Check sheet for the modelled part. Datum: model origin and axes. Units: mm. A direction names the side the tool comes from. Coordinates: 2 decimals unless noted, no trailing zeros. Order: outer loops, then holes, each group sorted by start corner. A loop starts at its lowest first (then second) coordinate and runs counter-clockwise, first axis right, second up. Notation, with made-up numbers: (42, 11.5) -> (89, 11.5) arc R26 ccw to (89, 26.5) -> close; hole circle Ø10 at (9, -31.75). An arc over 180 degrees is marked (long way). Put each result on its own line as item: value. Start each with the question number.
```python
from build123d import *

# Parameters (mm, degrees)
F0_W     = 57.15
F0_H     = 63.5
F1_DEPTH = 44.45
F2_W     = 22.225
F2_H     = 19.05
F3_DEPTH = 12.7
F4_W     = 19.05
F4_H     = 12.7
F5_DEPTH = 63.501


with BuildPart() as f1:
    # F0 (on Front) → F1 (new body)
    with BuildSketch(Plane.XZ):
        Rectangle(F0_W, F0_H)
    extrude(amount=F1_DEPTH)

    # F2 (on face) → F3 (join)
    with BuildSketch(Plane(origin=(0, 0, 0), x_dir=(-1, 0, 0), z_dir=(0, 1, 0))):
        with Locations((-39.6875, -22.225)):
            Rectangle(F2_W, F2_H)
    extrude(amount=-F3_DEPTH)

    # F4 (on face) → F5 (cut, through all)
    with BuildSketch(Plane.XY.offset(31.75)):
        with Locations((3.175, -38.1)):
            Rectangle(F4_W, F4_H)
    extrude(amount=-F5_DEPTH, mode=Mode.SUBTRACT)


solid = f1.part
```
1) Mould release check, pull along X, two halves, no side actions. Record for faces 4 (the flat face through (12.7, -38, 0)), 5 (the flat face through (50.8, -6, -22)), 6 (the flat face through (21, -44.45, 0)), 7 (the flat face through (-6.35, -38, 0)): +X half, -X half, draft (parallel to the pull), parting line (faces both ways), or undercut.
2) Sectioned sample at D-D (x = 32.5). Record the boundary of the cut face in (y, z).
3) Scan lines: line 1 along X through (y, z) = (-36, -24) (3 decimals); line 2 along X through (y, z) = (-28.5, -16.5) (3 decimals); line 3 along Y through (x, z) = (-5, -1). Record each from-to range of solid material in increasing order. Write a range as [from, to].
4) Gauge pin test, flat ends, axial feed: pin 1 (9.5 mm diameter, centred on x = 0.5, z = -4.5, fed in from -Y); pin 2 (3 mm diameter, centred on x = 30.5, y = -32, fed in from +Z); pin 3 (1 mm diameter, centred on y = -33, z = -13.5, fed in from +X) (3 decimals); pin 4 (14 mm diameter, centred on x = 39.5, y = -5.5, fed in from +Z). Record the tip position at first contact, or that the pin passes through.
5) Sectioned sample at B-B (z = 7). Record the boundary of the cut face in (x, y) (3 decimals).
6) Access from +Z, -Z, +X, -X, +Y, -Y to the whole of each face (thin tool, end or side, straight path). Record for faces 1 (the flat face through (40, -12.7, -22)), 2 (the flat face through (3, -31.75, 0)), 3 (the flat face through (40, -6, -12.7)).
7) Sectioned sample at C-C (y = -6). Record the boundary of the cut face in (x, z) (3 decimals), plus the area to 3 significant figures.
8) Sectioned sample at A-A (y = -33). Record the boundary of the cut face in (x, z) (3 decimals), plus the area to 3 significant figures.
Entries:
1. face 4: undercut
1. face 5: +X half
1. face 6: draft
1. face 7: undercut
2. outline: (-12.7, -31.75) -> (0, -31.75) -> (0, -12.7) -> (-12.7, -12.7) -> close
3. line 1: x = [-28.575, -6.35], [12.7, 28.575]
3. line 2: x = [-28.575, 28.575]
3. line 3: y = [-31.75, 0]
4. pin 1: stops at y = -31.75
4. pin 2: passes through
4. pin 3: stops at x = 28.575
4. pin 4: stops at z = -12.7
5. outline: (-28.575, -44.45) -> (-6.35, -44.45) -> (-6.35, -31.75) -> (12.7, -31.75) -> (12.7, -44.45) -> (28.575, -44.45) -> (28.575, 0) -> (-28.575, 0) -> close
6. face 1: +Z, -Z, +X, -Y
6. face 2: +Z, -Z, -Y
6. face 3: +Z, +X, +Y, -Y
7. outline: (-28.575, -31.75) -> (50.8, -31.75) -> (50.8, -12.7) -> (28.575, -12.7) -> (28.575, 31.75) -> (-28.575, 31.75) -> close
7. area: 4,050 mm2
8. outline: (-28.575, -31.75) -> (-6.35, -31.75) -> (-6.35, 31.75) -> (-28.575, 31.75) -> close; (12.7, -31.75) -> (28.575, -31.75) -> (28.575, 31.75) -> (12.7, 31.75) -> close
8. area: 2,420 mm2
